```python
from build123d import *

# Parameters (mm, degrees)
SKETCH1_R               = 4.85
BOSS_EXTRUDE1_DEPTH     = 224.6937
CUT_EXTRUDE1_DEPTH      = 225.798362582
CUT_EXTRUDE1_DEPTH_BACK = 225.798362582
SKETCH2_R               = 1.25
SCALE1_SCALE            = 1.5


with BuildPart() as part:
    # Sketch1 → Boss-Extrude1 (new body)
    with BuildSketch(Plane(origin=(0, 0, 0), x_dir=(0, 0, -1), z_dir=(1, 0, 0))):
        with Locations(Location((0, 0, 0), (0, 0, 180))):
            Circle(SKETCH1_R)
    extrude(amount=BOSS_EXTRUDE1_DEPTH)

    # Sketch2 → Cut-Extrude1 (cut, two sides: drawn at the far end of the back side and taken through both)
    with BuildSketch(Plane(origin=(0, 0, 0), x_dir=(1, 0, 0), z_dir=(0, 1, 0)).offset(-CUT_EXTRUDE1_DEPTH_BACK)):
        with Locations(Location((2.5, 0, 0), (0, 0, 270))):
            Circle(SKETCH2_R)
    extrude(amount=CUT_EXTRUDE1_DEPTH + CUT_EXTRUDE1_DEPTH_BACK, mode=Mode.SUBTRACT)


with BuildPart() as part_1:
    # Scale1: scaled about (112.660192286, 0, 1.805e-06)
    add(part.part.scale(SCALE1_SCALE).moved(Location((-56.330096143, 0, -9.03e-07))))


solid = part_1.part
```
Source: CAD feature listing. Evaluate the final solid. Frame: model axes, mm. Round coordinates to 2 decimals unless told otherwise and drop trailing zeros. Loops run counter-clockwise (first coordinate to the right, second up) from the corner with the lowest first, then second, coordinate; pieces in that order, holes last.
(1) Section query B-B (x = 234). Output: boundary loops of the cut face in (y, z) (3 decimals).
From the geometry:
outline: circle Ø14.55 at (0, 0)
(2) Section query A-A (y = 2.75). Output: boundary loops of the cut face in (x, z) (3 decimals).
From the geometry:
outline: (-56.33, -6.735) - (280.71, -6.735) - (280.71, 6.735) - (-56.33, 6.735) - close; hole circle Ø3.75 at (-52.58, 0)
(3) Material intervals for probe 1 along X at (y, z) = (-1, 0); probe 2 along Y at (x, z) = (218.5, -0.25); probe 3 along X at (y, z) = (-4.25, -1.25), sorted ascending.
From the geometry:
probe 1: x = -56.33 to -54.46, -50.71 to 280.71
probe 2: y = -7.27 to 7.27
probe 3: x = -56.33 to -53.98, -51.18 to 280.71
(4) Contact query for flat-ended pins moving along their axis: pin 1 Ø4 at (x, y) = (90, -1.5) entering from -Z (3 decimals); pin 2 Ø1 at (x, z) = (189.5, 3.5) entering from -Y; pin 3 Ø1 at (x, z) = (227.5, 5.5) entering from +Y; pin 4 Ø2 at (x, z) = (-52.58, 0) entering from +Y. Output: stop coordinate, or through.
From the geometry:
pin 1: stops at z = -7.275
pin 2: stops at y = -6.63
pin 3: stops at y = 5.28
pin 4: passes through
